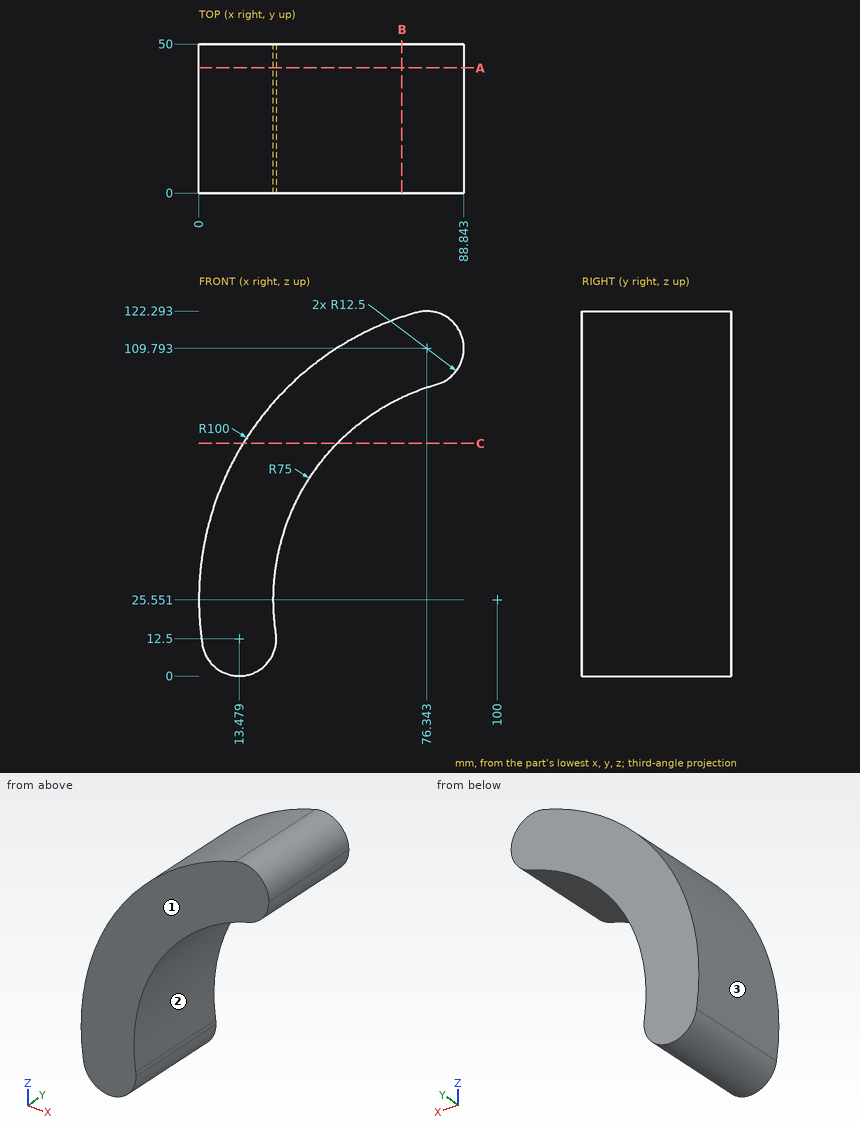
Print and shaded views of the part. All mm, measured from the part's lowest x, y and z. Coordinates: 2 decimals unless noted, no trailing zeros. Order: outer loops, then holes, each group sorted by start corner. A loop starts at its lowest first (then second) coordinate and runs counter-clockwise, first axis right, second up.
(1) Slice it at C-C, the plane z = 78. Write the cut outline in (x, y).
Check sheet entries:
outline: (14.86, 0) - (46.39, 0) - (46.39, 50) - (14.86, 50) - close
(2) Pin check, flat tips, straight feed: pin 1 Ø6 at (y, z) = (15, 35.5) entering from +X; pin 2 Ø8 at (y, z) = (38.5, 101) entering from -X (1 decimal); pin 3 Ø1 at (x, y) = (42.5, 8) entering from -Z. Stop position of each tip, or through.
Check sheet entries:
pin 1: stops at x = 26.13
pin 2: stops at x = 30
pin 3: stops at z = 73.1
(3) Slice it at A-A, the plane y = 42. Write the cut outline in (x, z) (1 decimal).
Check sheet entries:
outline: (1.1, 10.6) arc R12.5 ccw to (25.8, 14.4) arc R75 cw to (79.7, 97.8) arc R12.5 ccw to (73, 121.8) arc R100 ccw to start
(4) Pull direction X, two halves, no side cores. Call the marked faces 1, 2 and 3: pulls with the +X half, pulls with the -X half, needs draft (parallel to the pull), parting line crosses it, or undercut.
Check sheet entries:
face 1: needs draft
face 2: pulls with the +X half
face 3: pulls with the -X half
(5) Slice it at B-B, the plane x = 68. Write the cut outline in (y, z).
Check sheet entries:
outline: (0, 93.38) - (50, 93.38) - (50, 120.29) - (0, 120.29) - close
(6) Probe L1, parallel to X at y = 41.5, z = 24.5 (1 decimal); L2, parallel to Z at x = 48, y = 22; L3, parallel to X at y = 10, z = 116.5 (1 decimal). List the from-to ranges inside material, lowest first.
Check sheet entries:
L1: x = 0 to 25
L2: z = 79.6 to 110.97
L3: x = 58.4 to 86.9
